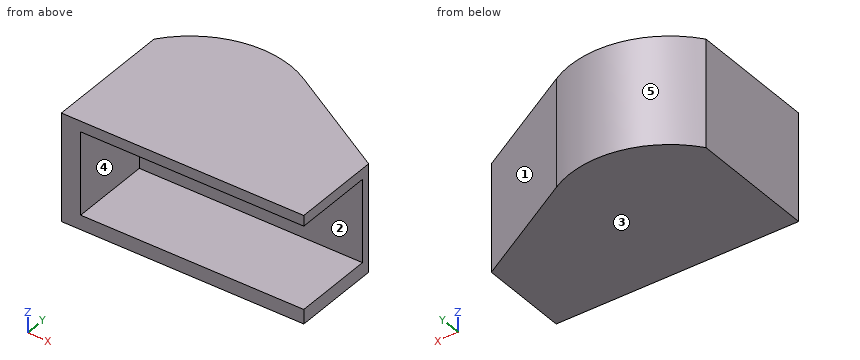
```python
from build123d import *

# Parameters (mm, degrees)
F1_DEPTH = 25.4
F2_W     = 52.6
F2_H     = 19.5
F3_DEPTH = 19


with BuildPart() as f1:
    # F0 (on Top) → F1 (new body)
    with BuildSketch(Plane.XY):
        with BuildLine():
            Line((0, 30), (0, 0))
            Line((0, 0), (57.15, 0))
            Line((57.15, 0), (57.15, 21))
            Line((57.15, 21), (30.746157, 36.244266))
            ThreePointArc((30.746157, 36.244266), (14.190828, 38.943421), (0, 30))
        make_face()
    extrude(amount=F1_DEPTH)

    # F2 (on face) → F3 (cut)
    with BuildSketch(Plane.XZ):
        with Locations((30.85, 13.15)):
            Rectangle(F2_W, F2_H)
    extrude(amount=-F3_DEPTH, mode=Mode.SUBTRACT)


solid = f1.part
```
Geometry check sheet. Reference: the model listing, model coordinates, mm. Face numbers are marked on the shaded views. A direction names the side the tool comes from. Coordinates: 2 decimals unless noted, no trailing zeros. Write each loop counter-clockwise with the first axis right and the second up, starting at its lowest first coordinate (ties: lowest second). Pieces come first, ordered by that corner, then holes. Notation, with made-up numbers: M 48.25,-9.75 L 92.25,-9.75 A34 cw 92.25,23.25 Z; hole C -16,22.5 d9. An arc over 180 degrees is marked long. Use one line per item in the form item = value. Start each with the question number.
1) Go/stop test with flat-tipped pins: pin 1 Ø8 at (x, z) = (14.5, 19) entering from +Y; pin 2 Ø2 at (x, z) = (26.5, 3) entering from +Y; pin 3 Ø9.5 at (y, z) = (7.5, 17.5) entering from +X. Record where each tip stops, or that it passes through.
2) Thickness scan on probe 1 along Z at (x, y) = (16, 5); probe 2 along X at (y, z) = (4, 8.5); probe 3 along X at (y, z) = (37, 15). Record the ranges inside material, lowest first. Write a range as from..to.
3) Section check C-C on x = 23.5. Enter the section's corners in (y, z), and give its area (3 significant figures).
4) Release check for a two-part mould opening along Z. For the marked faces 3, 4 and 5 record: pulls with the +Z half, pulls with the -Z half, needs draft (parallel to the pull), parting line crosses it, or undercut.
5) Section check D-D on y = 24.5. Enter the section's corners in (x, z).
6) Set-up check for the marked faces 1 and 2: record each of +Z, -Z, +X, -X, +Y, -Y from which the full face is reachable in a straight line by a thin tool's end or side.
7) Section check A-A on z = 21.75. Enter the section's corners in (x, y).
8) Section check B-B on y = 15. Enter the section's corners in (x, z).
Responses:
q1.pin_1 = 39.41
q1.pin_2 = 38.48
q1.pin_3 = 4.55
q2.probe_1 = 0..3.4, 22.9..25.4
q2.probe_2 = 0..4.55
q2.probe_3 = 8.48..29.33
q3.outline = M 0,0 L 38.97,0 L 38.97,25.4 L 0,25.4 L 0,22.9 L 19,22.9 L 19,3.4 L 0,3.4 Z
q3.area = 619 mm2
q4.face_3 = pulls with the -Z half
q4.face_4 = undercut
q4.face_5 = needs draft
q5.outline = M 0,0 L 51.09,0 L 51.09,25.4 L 0,25.4 Z
q6.face_1 = +Z, -Z, +X, +Y
q6.face_2 = +X, -Y
q7.outline = M 0,0 L 4.55,0 L 4.55,19 L 57.15,19 L 57.15,21 L 30.75,36.24 A23.68 ccw 0,30 Z
q8.outline = M 0,0 L 57.15,0 L 57.15,3.4 L 4.55,3.4 L 4.55,22.9 L 57.15,22.9 L 57.15,25.4 L 0,25.4 Z
